```python
from build123d import *

# Parameters (mm, degrees)
SKETCH_1_W            = 55
SKETCH_1_H            = 200
EXTRUDE_1_DEPTH       = 1
HOLE_WIZARD_M31_D     = 3.4
HOLE_WIZARD_M31_DEPTH = 5
HOLE_WIZARD_M31_TIP   = 1.021463052


with BuildPart() as part:
    # Эскиз1 → Бобышка-Вытянуть1 (new body)
    with BuildSketch(Plane.XY):
        with Locations((27.5, 100)):
            Rectangle(SKETCH_1_W, SKETCH_1_H)
    extrude(amount=EXTRUDE_1_DEPTH)

    # Отверстие с зазором M31
    with Locations(Plane(origin=(0, 0, 0), x_dir=(-1, 0, 0), z_dir=(0, 0, -1))):
        with Locations((-22, 175), (-22, 137.5), (-22, 100), (-22, 62.5), (-22, 25)):
            Hole(HOLE_WIZARD_M31_D / 2, depth=HOLE_WIZARD_M31_DEPTH)
            with Locations((0, 0, -(HOLE_WIZARD_M31_DEPTH + HOLE_WIZARD_M31_TIP / 2))):  # 118° drill point
                Cone(0, HOLE_WIZARD_M31_D / 2, HOLE_WIZARD_M31_TIP, mode=Mode.SUBTRACT)


solid = part.part
```
CAD build for the part. Positions are in the model's coordinates, mm. Give positions to 0.01 mm unless a question says otherwise; leave off trailing zeros. Loops run counter-clockwise (first coordinate to the right, second up) from the corner with the lowest first, then second, coordinate; pieces in that order, holes last. Notation, with made-up numbers: (-16.5, 72) - (-9.5, 72) arc R26 cw to (-9.5, 88) - close; hole circle Ø3 at (23.5, 87.25). An arc over 180 degrees is marked (long way). Put each result on its own line as item: value.
Q1. Probe line 1 along Y through (x, z) = (22, 0.3); line 2 along X through (y, z) = (100, 0.3); line 3 along X through (y, z) = (176, 0.3). List the from-to ranges inside material, lowest first.
Filled in:
line 1: y = 0 to 23.3, 26.7 to 60.8, 64.2 to 98.3, 101.7 to 135.8, 139.2 to 173.3, 176.7 to 200
line 2: x = 0 to 20.3, 23.7 to 55
line 3: x = 0 to 20.63, 23.37 to 55
Q2. Slice it at A-A (y = 100). Give the cut face in (x, z), plus the area to 3 significant figures.
Filled in:
outline: (0, 0) - (20.3, 0) - (20.3, 1) - (0, 1) - close; (23.7, 0) - (55, 0) - (55, 1) - (23.7, 1) - close
area: 51.6 mm²
Q3. Flat gauge pins, fed straight in: pin 1 (3 mm diameter, centred on x = 22, y = 25, fed in from -Z); pin 2 (10 mm diameter, centred on x = 36.5, y = 120, fed in from -Z). Where does each tip first touch, or does it go through?
Filled in:
pin 1: passes through
pin 2: stops at z = 0
Q4. Mould opens along X. For faces 1 (the face through (27, 101, 1)), 2 (the face through (22.914, 26.433, 0.507)) say: pulls with the +X half, pulls with the -X half, needs draft (parallel to the pull), parting line crosses it, or undercut.
Filled in:
face 1: needs draft
face 2: undercut
Q5. Slice it at B-B (x = 22). Give the cut face in (y, z), plus the area to 3 significant figures.
Filled in:
outline: (0, 0) - (23.3, 0) - (23.3, 1) - (0, 1) - close; (26.7, 0) - (60.8, 0) - (60.8, 1) - (26.7, 1) - close; (64.2, 0) - (98.3, 0) - (98.3, 1) - (64.2, 1) - close; (101.7, 0) - (135.8, 0) - (135.8, 1) - (101.7, 1) - close; (139.2, 0) - (173.3, 0) - (173.3, 1) - (139.2, 1) - close; (176.7, 0) - (200, 0) - (200, 1) - (176.7, 1) - close
area: 183 mm²
